from build123d import *

# Parameters (mm, degrees)
SKETCH_A01_1_R     = 6.85
EXTRUDE1_DEPTH     = 100
SKETCH1_W          = 6.892084618
SKETCH1_H          = 1.884433334
CUT_EXTRUDE1_DEPTH = 101


with BuildPart() as part:
    # Sketch A01-1 → Extrude1 (new body)
    with BuildSketch(Plane.XY):
        Polygon((-23.5, 4), (-25, 4), (-25, 25), (-4, 25), (-4, 23.349803168), (-5, 23.349803168), (-5, 22.349803168), (-4, 22.349803168), (-4, 21), (-8, 21), (-8, 23.5), (-11, 23.5), (-11, 21), (-11, 16.5), (-9.5, 16.5), (-9.5, 15.863961), (-3.78206785, 10.14602885), (3.78206785, 10.14602885), (9.5, 15.863961), (9.5, 16.5), (11, 16.5), (11, 21), (11, 23.5), (8, 23.5), (8, 21), (4, 21), (4, 22.349803168), (5, 22.349803168), (5, 23.349803168), (4, 23.349803168), (4, 25), (25, 25), (25, 4), (23.5, 4), (23.5, 5), (22.5, 5), (22.5, 4), (21, 4), (21, 8), (23.5, 8), (23.5, 11), (21, 11), (16.5, 11), (16.5, 9.5), (15.863961, 9.5), (10.14602885, 3.78206785), (10.14602885, -3.78206785), (15.863961, -9.5), (16.5, -9.5), (16.5, -11), (21, -11), (23.5, -11), (23.5, -8), (21, -8), (21, -4), (22.5, -4), (22.5, -5), (23.5, -5), (23.5, -4), (25, -4), (25, -25), (4, -25), (4, -23.349803168), (5, -23.349803168), (5, -22.349803168), (4, -22.349803168), (4, -21), (8, -21), (8, -23.5), (11, -23.5), (11, -21), (11, -16.5), (9.5, -16.5), (9.5, -15.863961), (3.78206785, -10.14602885), (-3.78206785, -10.14602885), (-9.5, -15.863961), (-9.5, -16.5), (-11, -16.5), (-11, -21), (-11, -23.5), (-8, -23.5), (-8, -21), (-4, -21), (-4, -22.349803168), (-5, -22.349803168), (-5, -23.349803168), (-4, -23.349803168), (-4, -25), (-25, -25), (-25, -4), (-23.5, -4), (-23.5, -5), (-22.5, -5), (-22.5, -4), (-21, -4), (-21, -8), (-23.5, -8), (-23.5, -11), (-21, -11), (-16.5, -11), (-16.5, -9.5), (-15.863961, -9.5), (-10.14602885, -3.78206785), (-10.14602885, 3.78206785), (-15.863961, 9.5), (-16.5, 9.5), (-16.5, 11), (-21, 11), (-23.5, 11), (-23.5, 8), (-21, 8), (-21, 4), (-22.5, 4), (-22.5, 5), (-23.5, 5), align=None)
        Circle(SKETCH_A01_1_R, mode=Mode.SUBTRACT)
        with BuildLine():
            Line((-23.5, 23.5), (-23.5, 12.5))
            Line((-23.5, 12.5), (-15, 12.5))
            Line((-15, 12.5), (-15, 10.757359344))
            Line((-15, 10.757359344), (-8.121320334, 3.878679677))
            ThreePointArc((-8.121320334, 3.878679677), (-6.363961031, 6.363961031), (-3.878679677, 8.121320334))
            Line((-3.878679677, 8.121320334), (-10.757359344, 15))
            Line((-10.757359344, 15), (-12.5, 15))
            Line((-12.5, 15), (-12.5, 23.5))
            Line((-12.5, 23.5), (-23.5, 23.5))
        make_face(mode=Mode.SUBTRACT)
        with BuildLine():
            Line((10.757359344, 15), (12.5, 15))
            Line((12.5, 15), (12.5, 23.5))
            Line((12.5, 23.5), (23.5, 23.5))
            Line((23.5, 23.5), (23.5, 12.5))
            Line((23.5, 12.5), (15, 12.5))
            Line((15, 12.5), (15, 10.757359344))
            Line((15, 10.757359344), (8.121320334, 3.878679677))
            ThreePointArc((8.121320334, 3.878679677), (6.363961031, 6.363961031), (3.878679677, 8.121320334))
            Line((3.878679677, 8.121320334), (10.757359344, 15))
        make_face(mode=Mode.SUBTRACT)
        with BuildLine():
            Line((23.5, -23.5), (23.5, -12.5))
            Line((23.5, -12.5), (15, -12.5))
            Line((15, -12.5), (15, -10.757359344))
            Line((15, -10.757359344), (8.121320334, -3.878679677))
            ThreePointArc((8.121320334, -3.878679677), (6.363961031, -6.363961031), (3.878679677, -8.121320334))
            Line((3.878679677, -8.121320334), (10.757359344, -15))
            Line((10.757359344, -15), (12.5, -15))
            Line((12.5, -15), (12.5, -23.5))
            Line((12.5, -23.5), (23.5, -23.5))
        make_face(mode=Mode.SUBTRACT)
        with BuildLine():
            Line((-10.757359344, -15), (-12.5, -15))
            Line((-12.5, -15), (-12.5, -23.5))
            Line((-12.5, -23.5), (-23.5, -23.5))
            Line((-23.5, -23.5), (-23.5, -12.5))
            Line((-23.5, -12.5), (-15, -12.5))
            Line((-15, -12.5), (-15, -10.757359344))
            Line((-15, -10.757359344), (-8.121320334, -3.878679677))
            ThreePointArc((-8.121320334, -3.878679677), (-6.363961031, -6.363961031), (-3.878679677, -8.121320334))
            Line((-3.878679677, -8.121320334), (-10.757359344, -15))
        make_face(mode=Mode.SUBTRACT)
    extrude(amount=-EXTRUDE1_DEPTH)

    # Sketch1 → Cut-Extrude1 (cut, through all)
    with BuildSketch(Plane.XY):
        with Locations((0.028776834, 6.878949495)):
            Rectangle(SKETCH1_W, SKETCH1_H)
    extrude(amount=-CUT_EXTRUDE1_DEPTH, mode=Mode.SUBTRACT)


solid = part.part
Source: CAD feature listing. Evaluate the final solid. Frame: model axes, mm. A direction names the side the tool comes from. Coordinates: 2 decimals unless noted, no trailing zeros. Loops run counter-clockwise (first coordinate to the right, second up) from the corner with the lowest first, then second, coordinate; pieces in that order, holes last. Notation, with made-up numbers: (39, 10.5) - (95, 10.5) arc R28 ccw to (95, 33.5) - close; hole circle Ø8 at (50, -36.5). An arc over 180 degrees is marked (long way). One line per item, written item: value. Start each with the question number.
1. Section B-B (y = 0). Return the cut outline in (x, z), and give its area (3 significant figures).
2. Ray query, L1, parallel to Y at x = 23, z = -80; L2, parallel to X at y = -16, z = -27; L3, parallel to Y at x = -18.5, z = -34. Return the intervals inside material, ascending.
3. Section C-C (x = -18). Return the cut outline in (y, z).
4. Section A-A (x = 0). Return the cut outline in (y, z).
5. Mould query, pull axis Y, two halves, no side actions, for faces 3 (the flat face through (25, 15, -49)), 4 (the flat face through (-23.5, -18, -49)), 5 (the flat face through (-14, -25, -49)). Classes: pulls with the +Y half, pulls with the -Y half, needs draft (parallel to the pull), parting line crosses it, or undercut.
6. Contact query for flat-ended pins moving along their axis: P1, Ø3, axis at x = 12, y = 10, coming from the -Z side; P2, Ø1, axis at x = 2, z = -73.5, coming from the -Y side. Output: stop coordinate, or through.
7. Set-up query: faces 1 (the flat face through (-12.5, 19, -49)), 2 (the flat face through (6, 6, 0)). Return all of +Z, -Z, +X, -X, +Y, -Y with unobstructed straight access to the full face (end or side cutting, diameter ignored); none if empty.
Verdict:
1. outline: (-10.15, -100) - (-6.85, -100) - (-6.85, 0) - (-10.15, 0) - close; (6.85, -100) - (10.15, -100) - (10.15, 0) - (6.85, 0) - close
1. area: 659 mm2
2. L1: y = -25 to -23.5, -12.5 to -11, -8 to -5, 5 to 8, 11 to 12.5, 23.5 to 25
2. L2: x = -25 to -23.5, -12.5 to -9.5, 9.5 to 12.5, 23.5 to 25
2. L3: y = -25 to -23.5, -12.5 to -11, 11 to 12.5, 23.5 to 25
3. outline: (-25, -100) - (-23.5, -100) - (-23.5, 0) - (-25, 0) - close; (-12.5, -100) - (-11, -100) - (-11, 0) - (-12.5, 0) - close; (11, -100) - (12.5, -100) - (12.5, 0) - (11, 0) - close; (23.5, -100) - (25, -100) - (25, 0) - (23.5, 0) - close
4. outline: (-10.15, -100) - (-6.85, -100) - (-6.85, 0) - (-10.15, 0) - close; (7.82, -100) - (10.15, -100) - (10.15, 0) - (7.82, 0) - close
5. face 3: needs draft
5. face 4: undercut
5. face 5: pulls with the -Y half
6. P1: passes through
6. P2: stops at y = -10.15
7. face 1: +Z, -Z
7. face 2: +Z, +X, -X, +Y, -Y
